Design review of the part built by this model. Coordinates are the model's own, in mm. Give positions to 0.01 mm unless a question says otherwise; leave off trailing zeros. Write each loop counter-clockwise with the first axis right and the second up, starting at its lowest first coordinate (ties: lowest second). Pieces come first, ordered by that corner, then holes. Notation, with made-up numbers: (-15.5, -4) -> (-9.5, -4) arc R27 cw to (-9.5, 30) -> close; hole circle Ø9 at (-2, -28.5). An arc over 180 degrees is marked (long way). Use CSV: the item, a comma, the result in double quotes.
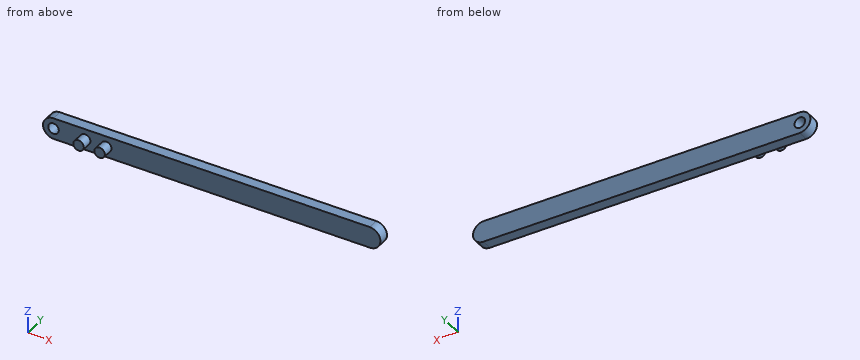
```python
from build123d import *

# Parameters (mm, degrees)
SKETCH1_R           = 2.5
BOSS_EXTRUDE1_DEPTH = 5
SKETCH2_R           = 2.5
BOSS_EXTRUDE2_DEPTH = 10


with BuildPart() as part:
    # Sketch1 → Boss-Extrude1 (new body)
    with BuildSketch(Plane(origin=(0, 0, 0), x_dir=(1, 0, 0), z_dir=(0, 1, 0))):
        with BuildLine():
            Line((-14.504443595, 6.706697569), (135.495556405, 4.691342482))
            ThreePointArc((135.495556405, 4.691342482), (140.42793273, -0.375378724), (135.361211524, -5.30775505))
            Line((135.361211524, -5.30775505), (-14.638788476, -3.292399963))
            ThreePointArc((-14.638788476, -3.292399963), (-19.571164802, 1.774321243), (-14.504443595, 6.706697569))
        make_face()
        with Locations(Location((-14.571616036, 1.707148803, 0), (0, 0, 270))):
            Circle(SKETCH1_R, mode=Mode.SUBTRACT)
    extrude(amount=BOSS_EXTRUDE1_DEPTH)

    # Sketch2 → Boss-Extrude2 (add)
    with BuildSketch(Plane(origin=(0, 5, 0), x_dir=(1, 0, 0), z_dir=(0, 1, 0))):
        with Locations(Location((0.428383964, 1.505613294, 0), (0, 0, 270))):
            Circle(SKETCH2_R)
        with Locations(Location((10.428383964, 1.371256288, 0), (0, 0, 270))):
            Circle(SKETCH2_R)
    extrude(amount=-BOSS_EXTRUDE2_DEPTH)


solid = part.part
```
(1) Take a section at C-C (y = 2.75). Write out the cut boundary in (x, z).
Established:
outline,"(-14.64, 3.29) arc R5 ccw to (-14.5, -6.71) -> (135.5, -4.69) arc R5 ccw to (135.36, 5.31) -> close; hole circle Ø5 at (-14.57, -1.71)"
(2) Clearance check with flat-ended pins moving along their axes: pin 1 (1.5 mm diameter, centred on x = 37.5, z = -1, fed in from -Y); pin 2 (6 mm diameter, centred on x = -14.57, z = -1.71, fed in from +Y); pin 3 (4 mm diameter, centred on x = 27, y = -3, fed in from -Z); pin 4 (1.5 mm diameter, centred on y = -2.5, z = -2.5, fed in from -X). State where each tip first meets the part, or that it passes through.
Established:
pin 1,"stops at y = 0"
pin 2,"stops at y = 5"
pin 3,"passes through"
pin 4,"stops at x = -2.06"
(3) For line 1 along Y through (x, z) = (29, -1.5); line 2 along X through (y, z) = (-2, -0.25); line 3 along X through (y, z) = (-2.25, 0), list the stretches that pass through material, from the lowest coordinate up. Write a range as [from, to].
Established:
line 1,"y = [0, 5]"
line 2,"x = [-1.73, 2.59], [8.19, 12.66]"
line 3,"x = [-1.57, 2.42], [8.34, 12.52]"
(4) Take a section at D-D (x = 46). Write out the cut boundary in (y, z), then the cut area to 3 significant figures.
Established:
outline,"(0, -5.89) -> (5, -5.89) -> (5, 4.11) -> (0, 4.11) -> close"
area,"50.0 mm2"
(5) Take a section at B-B (y = -3). Write out the cut boundary in (x, z).
Established:
outline,"circle Ø5 at (0.43, -1.51); circle Ø5 at (10.43, -1.37)"
(6) Take a section at A-A (z = -2.5). Write out the cut boundary in (x, y), then the cut area to 3 significant figures.
Established:
outline,"(-19.51, 0) -> (-16.94, 0) -> (-16.94, 5) -> (-19.51, 5) -> close; (-12.2, 0) -> (-1.87, 0) -> (-1.87, -5) -> (2.72, -5) -> (2.72, 0) -> (8.2, 0) -> (8.2, -5) -> (12.66, -5) -> (12.66, 0) -> (139.57, 0) -> (139.57, 5) -> (-12.2, 5) -> close"
area,"817 mm2"
